Read the model definition and answer for the solid it produces. Units are mm, in the model's axes. Face numbers are marked on the shaded views. Give positions to 0.01 mm unless a question says otherwise; leave off trailing zeros. Loops run counter-clockwise (first coordinate to the right, second up) from the corner with the lowest first, then second, coordinate; pieces in that order, holes last. Notation, with made-up numbers: (-10, -13.75) -> (30, -13.75) arc R28 cw to (30, 9.25) -> close; hole circle Ø5 at (10.25, -31). An arc over 180 degrees is marked (long way). Answer as CSV lines item,"result". Start each with the question number.
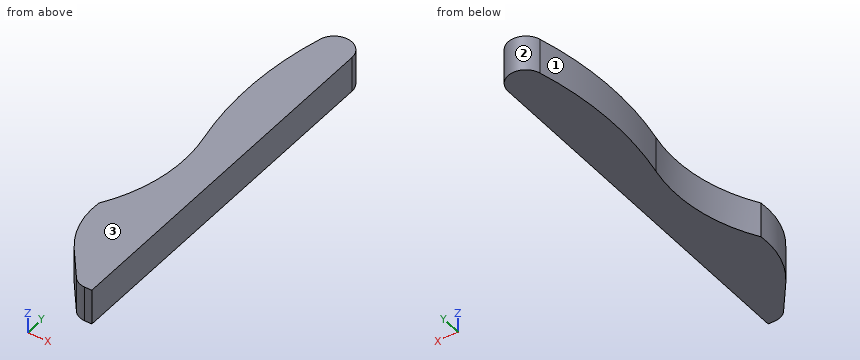
```python
from build123d import *

# Parameters (mm, degrees)
PAD_DEPTH = 10


with BuildPart() as part:
    # Sketch → Pad (new body)
    with BuildSketch(Plane.XY):
        with BuildLine():
            Line((0, 0), (0, -104))
            Line((0, -104), (-2, -104))
            ThreePointArc((-5.547641, -102.268437), (-3.973833, -103.544006), (-2, -104))
            Line((-5.547641, -102.268437), (-12, -94))
            ThreePointArc((-17, -77), (-16.119734, -85.976392), (-12, -94))
            ThreePointArc((-17, -77), (-10.720846, -60.862897), (-11, -43.549436))
            ThreePointArc((-9.829475, 1.29467), (-13.070868, -21.058052), (-11, -43.549436))
            ThreePointArc((0, 0), (-4.347074, 4.957185), (-9.829475, 1.29467))
        make_face()
    extrude(amount=PAD_DEPTH)


solid = part.part
```
(1) The mould has two halves that part along Y. Classify the marked faces 1, 2 and 3: pulls with the +Y half, pulls with the -Y half, needs draft (parallel to the pull), parting line crosses it, or undercut.
(2) Find the intervals of material crossed by line 1 along X through (y, z) = (-79, 2.5); line 2 along Y through (x, z) = (-6.5, 4); line 3 along Y through (x, z) = (-3.75, 6.5), in increasing order. Write a range as from..to.
(3) Find section C-C on x = -14.5. Write down the section's boundary in (y, z), then the cut area to 3 significant figures.
(4) Find section B-B on y = -63. Write down the section's boundary in (x, z).
(5) Each of these flat-tipped pins is pushed along its axis until it touches: P1, Ø6, axis at x = -9.5, z = 3, coming from the -Y side; P2, Ø5, axis at y = -23.5, z = 7.5, coming from the -X side; P3, Ø5, axis at y = -11, z = 4, coming from the -X side. Where does it stop, or does it pass through?
(6) Find section A-A on z = 2.5. Write down the section's boundary in (x, y).
Answer block:
1,face 1,"undercut"
1,face 2,"pulls with the +Y half"
1,face 3,"needs draft"
2,line 1,"x = -17.1..0"
2,line 2,"y = -101.05..4.77"
2,line 3,"y = -103.65..4.84"
3,outline,"(-90.06, 0) -> (-72.5, 0) -> (-72.5, 10) -> (-90.06, 10) -> close"
3,area,"176 mm2"
4,outline,"(-11.16, 0) -> (0, 0) -> (0, 10) -> (-11.16, 10) -> close"
5,P1,"stops at y = -101.05"
5,P2,"stops at x = -13.1"
5,P3,"stops at x = -12.57"
6,outline,"(-17, -77) arc R24.09 ccw to (-12, -94) -> (-5.55, -102.27) arc R4.5 ccw to (-2, -104) -> (0, -104) -> (0, 0) arc R5 ccw to (-9.83, 1.29) arc R96 ccw to (-11, -43.55) arc R45 cw to start"
